Autodesk Inventor part; units mm, degrees
ref_plane "YZ Plane" through (0, 0, 0) normal (1, 0, 0) x (0, 1, 0)
ref_plane "XZ Plane" through (0, 0, 0) normal (0, 1, 0) x (-1, 0, 0)
ref_plane "XY Plane" through (0, 0, 0) normal (0, 0, 1) x (1, 0, 0)
sketch "Sketch1" plane through (0, 0, 0) normal (0, 0, 1) x (1, 0, 0)
  line L0 (-25, -7.5) -> (25, -7.5)
  line L1 (25, -7.5) -> (25, 7.5)
  line L2 (25, 7.5) -> (-25, 7.5)
  line L3 (-25, 7.5) -> (-25, -7.5)
  line L4 (-25, -7.5) -> (25, 7.5) construction
  line L5 (25, -7.5) -> (-25, 7.5) construction
  point P0 (0, 0)
  dimension "d0" = 50
  dimension "d1" = 15
extrude "Extrusion1" add sketch "Sketch1" along normal blind 1.5
sketch "Sketch2" plane through (0, 0, 1.5) normal (0, 0, 1) x (1, 0, 0)
  circle A0 centre (-20, 0) radius 1.25
  line L0 (0, -11.9497) -> (0, 11.9497)
  circle A1 centre (20, 0) radius 1.25
  line L1 (-25, 7.5) -> (-25, -7.5)
  point P0 (0, 0)
  dimension "d4" = 2.5
  dimension "d5" = 5
extrude "Extrusion2" cut sketch "Sketch2" against normal up to next
fillet "Fillet1" radius 5 4 edges at (25, 7.5, 0.75) (25, -7.5, 0.75) (-25, -7.5, 0.75) (-25, 7.5, 0.75)
sketch "Sketch3" plane through (0, 0, 1.5) normal (0, 0, 1) x (1, 0, 0)
  line L0 (-10.4543, 4.2971) -> (11.6893, 4.2971) construction
  line L1 (11.6893, 4.2971) -> (11.6893, -4.6339) construction
  line L2 (11.6893, -4.6339) -> (-10.4543, -4.6339) construction
  line L3 (-10.4543, -4.6339) -> (-10.4543, 4.2971) construction
sketch "Sketch4" plane through (0, 0, 0) normal (0, 0, -1) x (-1, 0, 0)
  line L0 (-10.4543, 4.2971) -> (11.6893, 4.2971) construction
  line L1 (11.6893, 4.2971) -> (11.6893, -4.6339) construction
  line L2 (11.6893, -4.6339) -> (-10.4543, -4.6339) construction
  line L3 (-10.4543, -4.6339) -> (-10.4543, 4.2971) construction
sketch "Sketch5" plane through (0, 0, 0) normal (0, 0, -1) x (-1, 0, 0)
  circle A0 centre (20, 0) radius 1.25
  circle A1 centre (-20, 0) radius 1.25
  arc A2 (25, 2.5) -> (20, 7.5) centre (20, 2.5) ccw
  line L0 (-20, 7.5) -> (20, 7.5)
  arc A3 (-20, 7.5) -> (-25, 2.5) centre (-20, 2.5) ccw
  line L1 (-25, -2.5) -> (-25, 2.5)
  arc A4 (-25, -2.5) -> (-20, -7.5) centre (-20, -2.5) ccw
  line L2 (20, -7.5) -> (-20, -7.5)
  arc A5 (20, -7.5) -> (25, -2.5) centre (20, -2.5) ccw
  line L3 (25, 2.5) -> (25, -2.5)
  point P0 (0, 0)
equation "\"d0\" = l_label"
equation "\"d1\" = w_label"
equation "\"d4\" = r_labelscrew"
equation "\"d5\" = ro_labelscrew"
equation "\"d8\" = ro_labelscrew"
equation "\"wl_panel\" = 285"
equation "\"t_panel\" = 8"
equation "\"r_button\" = 8"
equation "\"l_stereo\" = 178"
equation "\"d_stereo\" = 177"
equation "\"w_label\" = 15"
equation "\"l_label\" = 50"
equation "\"r_labelscrew\" = 2.5"
equation "\"ro_labelscrew\" = 5"
equation "\"l_buttontobutton\" = 25"
equation "\"r_usboutlet\" = 29"
equation "\"l_fastener_button\" = 19"
properties part number "label" material "Stainless Steel"
Here's how the part is built. I have some questions about the finished solid (model axes, mm). Round coordinates to 2 decimals unless told otherwise and drop trailing zeros. Order: outer loops, then holes, each group sorted by start corner. A loop starts at its lowest first (then second) coordinate and runs counter-clockwise, first axis right, second up. Notation, with made-up numbers: (82, -6.5) -> (92, -6.5) arc R21 cw to (92, 11.5) -> close; hole circle Ø6 at (-38.5, 1). An arc over 180 degrees is marked (long way). Use a Markdown table: item, result. Add a question column.
(1) I need wall thicknesses on line 1 along Y through (x, z) = (-20, 0.6); line 2 along X through (y, z) = (-1, 0.35); line 3 along Y through (x, z) = (19, 1.05). Which ranges of each line are inside material? Lowest first, please.
(2) If we mould it in two halves opening along X, with no side actions, what happens to faces 1 (the face through (-18.845, -0.479, 0.76)), 2 (the face through (0, 0, 0)), 3 (the face through (-23.57, -6, 0.76))? For each: released by +X, released by -X, zero draft, split by the parting line, or undercut.
(3) Suppose I cut it at A-A, the plane z = 1.05. Please give me the cut outline in (x, y).
(4) Suppose I cut it at B-B, the plane y = 0. Please give me the cut outline in (x, z).
(5) For pin 1 Ø2 at (x, y) = (-20, 0) entering from +Z, with a flat end and sliding along its axis, tell me the tip position at first contact or that it passes through.
(6) Suppose I cut it at C-C, the plane y = -6. Please give me the cut outline in (x, z), and give its area (3 significant figures).
Verdict:
| question | item | result |
|---|---|---|
| 1 | line 1 | -7.5 to -1.25, 1.25 to 7.5 |
| 1 | line 2 | -25 to -20.75, -19.25 to 19.25, 20.75 to 25 |
| 1 | line 3 | -7.5 to -0.75, 0.75 to 7.5 |
| 2 | face 1 | undercut |
| 2 | face 2 | zero draft |
| 2 | face 3 | released by -X |
| 3 | outline | (-25, -2.5) arc R5 ccw to (-20, -7.5) -> (20, -7.5) arc R5 ccw to (25, -2.5) -> (25, 2.5) arc R5 ccw to (20, 7.5) -> (-20, 7.5) arc R5 ccw to (-25, 2.5) -> close; hole circle Ø2.5 at (-20, 0); hole circle Ø2.5 at (20, 0) |
| 4 | outline | (-25, 0) -> (-21.25, 0) -> (-21.25, 1.5) -> (-25, 1.5) -> close; (-18.75, 0) -> (18.75, 0) -> (18.75, 1.5) -> (-18.75, 1.5) -> close; (21.25, 0) -> (25, 0) -> (25, 1.5) -> (21.25, 1.5) -> close |
| 5 | pin 1 | through |
| 6 | outline | (-23.57, 0) -> (23.57, 0) -> (23.57, 1.5) -> (-23.57, 1.5) -> close |
| 6 | area | 70.7 mm2 |
